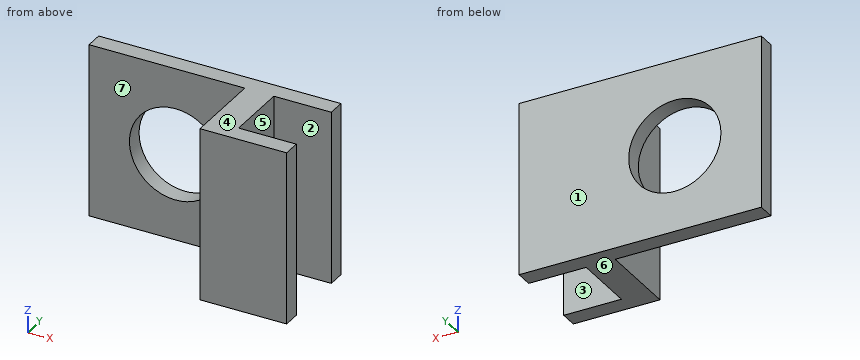
Autodesk Inventor part; units mm, degrees
ref_plane "YZ Plane" through (0, 0, 0) normal (1, 0, 0) x (0, 1, 0)
ref_plane "XZ Plane" through (0, 0, 0) normal (0, 1, 0) x (-1, 0, 0)
ref_plane "XY Plane" through (0, 0, 0) normal (0, 0, 1) x (1, 0, 0)
sketch "スケッチ1" plane through (0, 0, 0) normal (0, 1, 0) x (-1, 0, 0)
  line L0 (28.9798, 2.6849) -> (-13.0202, 2.6849)
  line L1 (-13.0202, 2.6849) -> (-13.0202, -27.3151)
  line L2 (-13.0202, -27.3151) -> (28.9798, -27.3151)
  line L3 (28.9798, -27.3151) -> (28.9798, 2.6849)
  circle A0 centre (13.9798, -12.3151) radius 8
  line L4 (-13.0202, 2.6849) -> (-3.0202, 2.6849)
  line L5 (-3.0202, 2.6849) -> (-3.0202, -27.3151)
  line L6 (-3.0202, -27.3151) -> (-13.0202, -27.3151)
  line L7 (-13.0202, -27.3151) -> (-13.0202, 2.6849)
  point P0 (0, 0)
  dimension "d0" = 16
  dimension "d1" = 30
  dimension "d2" = 15
  dimension "d3" = 15
  dimension "d4" = 15
  dimension "d5" = 27
  dimension "d6" = 10
  dimension "d7" = 9
extrude "押し出し1" add sketch "スケッチ1" along normal blind 3
sketch "スケッチ2" plane through (0, 0, 0) normal (0, -1, 0) x (1, 0, 0)
  line L0 (-28.9798, 2.6849) -> (13.0202, 2.6849)
  line L1 (13.0202, -27.3151) -> (-28.9798, -27.3151)
  line L2 (3.0499, 2.6849) -> (-1.9798, 2.6849)
  line L3 (-1.9798, 2.6849) -> (-1.9798, -27.3151)
  line L4 (-1.9798, -27.3151) -> (3.0499, -27.3151)
  line L5 (3.0499, -27.3151) -> (3.0499, 2.6849)
  circle A0 centre (-13.9798, -12.3151) radius 8
  point P0 (0, 0)
  dimension "d10" = 4
extrude "押し出し2" add sketch "スケッチ2" along normal blind 14 contours L0 L5 L1 L3
sketch "スケッチ3" plane through (3.0499, 0, 2.6849) normal (1, 0, 0) x (0, 0, -1)
  line L0 (0, -14) -> (30, -14)
  line L1 (30, -14) -> (0, -14)
  line L2 (0, -14) -> (0, -11)
  line L3 (0, -11) -> (30, -11)
  line L4 (30, -11) -> (30, -14)
  line L5 (0, 0) -> (30, 0)
  point P0 (2.6849, 0)
  dimension "d13" = 3
  dimension "d14" = 11
extrude "押し出し3" add sketch "スケッチ3" along normal blind 10
properties part number "emswparts"
Check sheet for the modelled part. Datum: model origin and axes. Units: mm. Face numbers are marked on the shaded views. A direction names the side the tool comes from. Coordinates: 2 decimals unless noted, no trailing zeros. Loops run counter-clockwise (first coordinate to the right, second up) from the corner with the lowest first, then second, coordinate; pieces in that order, holes last. Notation, with made-up numbers: (14, 36) -> (19, 36) arc R27 cw to (19, 65) -> close; hole circle Ø5 at (29.5, 27). An arc over 180 degrees is marked (long way). Answer in a Markdown table with one row per item.
1. Sectioned sample at C-C, the plane z = -0.5. Record the boundary of the cut face in (x, y), then the cut area to 3 significant figures.
Check values:
| item | result |
|---|---|
| outline | (-28.98, 0) -> (-1.98, 0) -> (-1.98, -14) -> (13.05, -14) -> (13.05, -11) -> (3.05, -11) -> (3.05, 0) -> (13.02, 0) -> (13.02, 3) -> (-28.98, 3) -> close |
| area | 226 mm2 |
2. Sectioned sample at B-B, the plane z = -13. Record the boundary of the cut face in (x, y), then the cut area to 3 significant figures.
Check values:
| item | result |
|---|---|
| outline | (-28.98, 0) -> (-21.95, 0) -> (-21.95, 3) -> (-28.98, 3) -> close; (-6.01, 0) -> (-1.98, 0) -> (-1.98, -14) -> (13.05, -14) -> (13.05, -11) -> (3.05, -11) -> (3.05, 0) -> (13.02, 0) -> (13.02, 3) -> (-6.01, 3) -> close |
| area | 179 mm2 |
3. Sectioned sample at A-A, the plane x = 10. Record the boundary of the cut face in (y, z), then the cut area to 3 significant figures.
Check values:
| item | result |
|---|---|
| outline | (-14, -27.32) -> (-11, -27.32) -> (-11, 2.68) -> (-14, 2.68) -> close; (0, -27.32) -> (3, -27.32) -> (3, 2.68) -> (0, 2.68) -> close |
| area | 180 mm2 |
4. Material ranges on line 1 along Y through (x, z) = (-6, -25.25); line 2 along X through (y, z) = (-9.5, -24); line 3 along X through (y, z) = (-12.5, -16), recorded low to high. Write a range as [from, to].
Check values:
| item | result |
|---|---|
| line 1 | y = [0, 3] |
| line 2 | x = [-1.98, 3.05] |
| line 3 | x = [-1.98, 13.05] |
5. Access from +Z, -Z, +X, -X, +Y, -Y to the whole of each face (thin tool, end or side, straight path). Record for the marked faces 5, 6 and 7.
Check values:
| item | result |
|---|---|
| face 5 | +Z, -Z, +X |
| face 6 | -Z, +X, -X, +Y, -Y |
| face 7 | +Z, -Z, -X, -Y |
6. Release check for a two-part mould opening along Y. For the marked faces 1, 2, 3 and 4 record: released by +Y, released by -Y, zero draft, split by the parting line, or undercut.
Check values:
| item | result |
|---|---|
| face 1 | released by +Y |
| face 2 | undercut |
| face 3 | undercut |
| face 4 | zero draft |
7. Go/stop test with flat-tipped pins: pin 1 (3.5 mm diameter, centred on y = -3.5, z = -12.5, fed in from +X); pin 2 (0.9 mm diameter, centred on y = 1.5, z = -11, fed in from +X); pin 3 (10 mm diameter, centred on x = -7.5, z = -20, fed in from -Y); pin 4 (10 mm diameter, centred on x = -11.5, y = -2, fed in from +Z). Record where each tip stops, or that it passes through.
Check values:
| item | result |
|---|---|
| pin 1 | stops at x = 3.05 |
| pin 2 | stops at x = 13.02 |
| pin 3 | stops at y = 0 |
| pin 4 | stops at z = 2.68 |
8. Sectioned sample at D-D, the plane y = 1. Record the boundary of the cut face in (x, z), then the cut area to 3 significant figures.
Check values:
| item | result |
|---|---|
| outline | (-28.98, -27.32) -> (13.02, -27.32) -> (13.02, 2.68) -> (-28.98, 2.68) -> close; hole circle Ø16 at (-13.98, -12.32) |
| area | 1,060 mm2 |
